Here's how the part is built. I have some questions about the finished solid (model axes, mm). A direction names the side the tool comes from. Give positions to 0.01 mm unless a question says otherwise; leave off trailing zeros. Loops run counter-clockwise (first coordinate to the right, second up) from the corner with the lowest first, then second, coordinate; pieces in that order, holes last.
Q1. Suppose I cut it at D-D (x = -1.5). List the corners of the cut face in (y, z) for me.
Q2. For faces 1 (the face through (12.496, -5.243, 1.972)), 2 (the face through (-22.132, -20, 2)), 3 (the face through (-18.286, -29.701, 2.028)), which set-ups out of +Z, -Z, +X, -X, +Y, -Y let a thin tool reach every point of the face, with its end or its side?
Q3. I need wall thicknesses on probe 1 along X at (y, z) = (-26, 3.8); probe 2 along X at (y, z) = (-20, 3.5); probe 3 along X at (y, z) = (-25.5, 3.3). Which ranges of each line are inside material? Lowest first, please.
Q4. I'm going to push flat-ended pins straight in: P1, Ø2, axis at y = -23.5, z = 2.5, coming from the +X side; P2, Ø1, axis at x = -7, z = 0.5, coming from the -Y side; P3, Ø1.2, axis at y = -17, z = 3, coming from the +X side. Where does each tip first touch, or does it pass through?
Q5. Thinking about a two-plate mould opening in Y: for faces 4 (the face through (17.132, -17, 2)), 5 (the face through (19.494, -29.794, 2.028)), 6 (the face through (22.132, -16, 2)), 7 (the face through (-17.845, -33.044, 1.972)), which applies, pulls with the +Y half, pulls with the -Y half, needs draft (parallel to the pull), parting line crosses it, or undercut?
Q6. Suppose I cut it at C-C (y = -29). List the corners of the cut face in (x, z) for me.
Q7. Suppose I cut it at A-A (y = -15). List the corners of the cut face in (x, z) for me, and give its area (3 significant figures).
```python
from build123d import *

# Parameters (mm, degrees)
SALIENTE_EXTRUIR4_DEPTH = 4
REDONDEO1_R             = 8
CROQUIS4_R              = 4
SALIENTE_EXTRUIR5_DEPTH = 4
CROQUIS5_R              = 2.1
CORTAR_EXTRUIR1_DEPTH   = 10
CROQUIS6_W              = 5
CROQUIS6_H              = 11
SALIENTE_EXTRUIR6_DEPTH = 4
REDONDEO2_R             = 2.5
CORTAR_EXTRUIR3_DEPTH   = 10
REDONDEO5_R             = 2
REDONDEO6_R             = 2


# Some blends are built 0.0001 mm under size
with BuildPart() as part:
    # Croquis3 → Saliente-Extruir4 (new body)
    with BuildSketch(Plane.XY):
        Polygon((-15.5, 0), (15.5, 0), (22.13230058, -4.473543228), (22.13230058, -22.795964517), (17.13230058, -22.795964517), (17.13230058, -7.795964517), (12.987112718, -5), (-12.987112718, -5), (-17.13230058, -7.795964517), (-17.13230058, -22.795964517), (-22.13230058, -22.795964517), (-22.13230058, -4.473543228), align=None)
    extrude(amount=SALIENTE_EXTRUIR4_DEPTH)

    # Redondeo1
    # the kernel refuses this fillet: 8 mm, written as the material it adds along each edge
    with BuildSketch(Plane(origin=(-12.987112718, -5, 0), x_dir=(1, 0, 0), z_dir=(0, 0, 1)), Plane(origin=(12.987112718, -5, 0), x_dir=(0.8290375725550433, -0.5591929034707446, 0), z_dir=(0, 0, 1))) as redondeo1_piece_1:
        with BuildLine():
            CenterArc((REDONDEO1_R * 0.305730681459, -REDONDEO1_R), REDONDEO1_R, 90, 34)
            Line((-REDONDEO1_R * 0.253462222012, -REDONDEO1_R * 0.170962427445), (0, 0))
            Line((0, 0), (REDONDEO1_R * 0.305730681459, 0))
        make_face()
    extrude(amount=4)
    with BuildSketch(Plane(origin=(-17.13230058, -7.795964517, 0), x_dir=(0.8290375725550426, 0.5591929034707452, 0), z_dir=(0, 0, 1)), Plane(origin=(17.13230058, -7.795964517, 0), x_dir=(0, -1, 0), z_dir=(0, 0, 1))) as redondeo1_piece_2:
        with BuildLine():
            CenterArc((REDONDEO1_R * 0.531709431661, -REDONDEO1_R), REDONDEO1_R, 90, 56)
            Line((-REDONDEO1_R * 0.297328140894, -REDONDEO1_R * 0.440807096529), (0, 0))
            Line((0, 0), (REDONDEO1_R * 0.531709431661, 0))
        make_face()
    extrude(amount=4)
    # the kernel refuses this fillet: 8 mm, written as the material it takes off along each edge
    with BuildSketch(Plane(origin=(22.13230058, -4.473543228, -10.634188633), x_dir=(-0.8290375725550431, 0.5591929034707448, 0), z_dir=(0, 0, 1))) as redondeo1_2_piece_1:
        with BuildLine():
            CenterArc((REDONDEO1_R * 0.531709431661, REDONDEO1_R), REDONDEO1_R, 214, 56)
            Line((-REDONDEO1_R * 0.297328140894, REDONDEO1_R * 0.440807096529), (0, 0))
            Line((0, 0), (REDONDEO1_R * 0.531709431661, 0))
        make_face()
    extrude(amount=25.268377266, mode=Mode.SUBTRACT)
    with BuildSketch(Plane(origin=(15.5, 0, -6.114613629), x_dir=(-1, 0, 0), z_dir=(0, 0, 1))) as redondeo1_2_piece_2:
        with BuildLine():
            CenterArc((REDONDEO1_R * 0.305730681459, REDONDEO1_R), REDONDEO1_R, 236, 34)
            Line((-REDONDEO1_R * 0.253462222012, REDONDEO1_R * 0.170962427445), (0, 0))
            Line((0, 0), (REDONDEO1_R * 0.305730681459, 0))
        make_face()
    extrude(amount=16.229227258, mode=Mode.SUBTRACT)
    with BuildSketch(Plane(origin=(-15.5, 0, -6.114613629), x_dir=(1, 0, 0), z_dir=(0, 0, 1))) as redondeo1_2_piece_3:
        with BuildLine():
            CenterArc((REDONDEO1_R * 0.305730681459, -REDONDEO1_R), REDONDEO1_R, 90, 34)
            Line((-REDONDEO1_R * 0.253462222012, -REDONDEO1_R * 0.170962427445), (0, 0))
            Line((0, 0), (REDONDEO1_R * 0.305730681459, 0))
        make_face()
    extrude(amount=16.229227258, mode=Mode.SUBTRACT)
    with BuildSketch(Plane(origin=(-22.13230058, -4.473543228, -10.634188633), x_dir=(0.8290375725550428, 0.5591929034707449, 0), z_dir=(0, 0, 1))) as redondeo1_2_piece_4:
        with BuildLine():
            CenterArc((REDONDEO1_R * 0.531709431661, -REDONDEO1_R), REDONDEO1_R, 90, 56)
            Line((-REDONDEO1_R * 0.297328140894, -REDONDEO1_R * 0.440807096529), (0, 0))
            Line((0, 0), (REDONDEO1_R * 0.531709431661, 0))
        make_face()
    extrude(amount=25.268377266, mode=Mode.SUBTRACT)

    # Croquis4 → Saliente-Extruir5 (add, through all)
    with BuildSketch(Plane.XY.offset(4)):
        with Locations((19.63230058, -25.795964517)):
            Circle(CROQUIS4_R)
    extrude(amount=-SALIENTE_EXTRUIR5_DEPTH)

    # Croquis5 → Cortar-Extruir1 (cut)
    with BuildSketch(Plane.XY.offset(4)):
        with Locations((19.63230058, -25.795964517)):
            Circle(CROQUIS5_R)
    extrude(amount=-CORTAR_EXTRUIR1_DEPTH, mode=Mode.SUBTRACT)

    # Croquis6 → Saliente-Extruir6 (add, through all)
    with BuildSketch(Plane.XY.offset(4)):
        with Locations((-19.63230058, -28.295964517)):
            Rectangle(CROQUIS6_W, CROQUIS6_H)
    extrude(amount=-SALIENTE_EXTRUIR6_DEPTH)

    # Redondeo2
    redondeo2_edges = [part.edges().sort_by_distance(p)[0] for p in [
        (-17.13230058, -33.795964517, 2),
        (-22.13230058, -33.795964517, 2),
    ]]
    fillet(redondeo2_edges, radius=REDONDEO2_R - 0.0001)  # a hair under: the kernel refuses the full size

    # Croquis8 → Cortar-Extruir3 (cut)
    with BuildSketch(Plane.XY.offset(4)):
        Polygon((-17.13230058, -31.156317686), (-19.139649056, -31.156317686), (-17.13230058, -27.735081186), align=None)
    extrude(amount=-CORTAR_EXTRUIR3_DEPTH, mode=Mode.SUBTRACT)

    # Redondeo5
    redondeo5_edges = [part.edges().sort_by_distance(p)[0] for p in [
        (-17.13230058, -27.735081186, 2),
    ]]
    fillet(redondeo5_edges, radius=REDONDEO5_R)

    # Redondeo6
    # the kernel refuses this fillet: 2 mm, written as the material it takes off along each edge
    with BuildSketch(Plane(origin=(-17.13230058, -31.156317686, 5.83619537), x_dir=(-1, 0, 0), z_dir=(0, 0, -1))) as redondeo6_piece_1:
        with BuildLine():
            CenterArc((0.734478148, -2), REDONDEO6_R, 90, 21.545444272)
            Line((0, -0.139746832), (-0.014689563, -0.102541768))
            ThreePointArc((-0.014689563, -0.102541768), (-0.04, -0.069873416), (-0.04, 0))
            Line((-0.04, 0), (0, 0.04))
            Line((0, 0.04), (0.734478148, 0.04))
            Line((0.734478148, 0.04), (0.734478148, 0))
        make_face()
    extrude(amount=7.672390741, mode=Mode.SUBTRACT)


solid = part.part
```
Solutions:
1. outline: (-5, 0) - (0, 0) - (0, 4) - (-5, 4) - close
2. face 1: +Z, -Z, -Y
2. face 2: +Z, -Z, -X, +Y, -Y
2. face 3: +Z, -Z
3. probe 1: x = -22.13 to -17.13, 15.64 to 17.54, 21.72 to 23.63
3. probe 2: x = -22.13 to -17.13, 17.13 to 22.13
3. probe 3: x = -22.13 to -17.13, 15.64 to 17.55, 21.71 to 23.62
4. P1: stops at x = 23.42
4. P2: stops at y = -5
4. P3: stops at x = 22.13
5. face 4: undercut
5. face 5: undercut
5. face 6: needs draft
5. face 7: pulls with the -Y half
6. outline: (-22.13, 0) - (-17.87, 0) - (-17.87, 4) - (-22.13, 4) - close; (17.24, 0) - (22.03, 0) - (22.03, 4) - (17.24, 4) - close
7. outline: (-22.13, 0) - (-17.13, 0) - (-17.13, 4) - (-22.13, 4) - close; (17.13, 0) - (22.13, 0) - (22.13, 4) - (17.13, 4) - close
7. area: 40.0 mm2
